Can you work these out from the model? Positions are in its coordinate system, mm. Give positions to 0.01 mm unless a question says otherwise; leave off trailing zeros. Order: outer loops, then holes, each group sorted by start corner. A loop starts at its lowest first (then second) coordinate and runs counter-clockwise, first axis right, second up. Notation, with made-up numbers: (44.5, 83) - (54.5, 83) arc R22 ccw to (54.5, 97) - close; hole circle Ø3 at (87.25, 3). An arc over 180 degrees is marked (long way). Return JSON: item names as keys, results as strings.
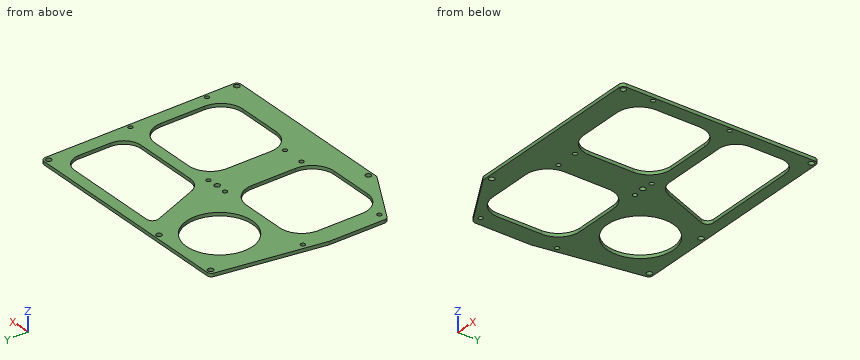
```python
from build123d import *

# Parameters (mm, degrees)
SKETCH_R   = 2.5
SKETCH_R_2 = 2
SKETCH_R_3 = 30.106081
PAD_DEPTH  = 3
FILLET_R   = 4


with BuildPart() as part:
    # Sketch → Pad (new body)
    with BuildSketch(Plane.XY.offset(30)):
        Polygon((162.56, -90.17), (-5.000233, -90.169747), (-56.898089, -60.365632), (-56.898089, -7.158878), (-41.241165, 90.17), (162.56, 90.17), align=None)
        with Locations((25.4, 86.106)):
            Circle(SKETCH_R, mode=Mode.SUBTRACT)
        with Locations((158.496, 86.106)):
            Circle(SKETCH_R, mode=Mode.SUBTRACT)
        with Locations((55.4, 10.106)):
            Circle(SKETCH_R, mode=Mode.SUBTRACT)
        with Locations((0.007, -86.11)):
            Circle(SKETCH_R, mode=Mode.SUBTRACT)
        with Locations((158.496, -86.106)):
            Circle(SKETCH_R, mode=Mode.SUBTRACT)
        with Locations((-36.83, 86.11)):
            Circle(SKETCH_R, mode=Mode.SUBTRACT)
        with Locations((159.06, -59.17)):
            Circle(SKETCH_R_2, mode=Mode.SUBTRACT)
        with Locations((159.059998, 10.83)):
            Circle(SKETCH_R_2, mode=Mode.SUBTRACT)
        with Locations((65.059998, 10.830006)):
            Circle(SKETCH_R_2, mode=Mode.SUBTRACT)
        with Locations((65.06, -59.169994)):
            Circle(SKETCH_R_2, mode=Mode.SUBTRACT)
        with Locations((45.06, -59.169992)):
            Circle(SKETCH_R_2, mode=Mode.SUBTRACT)
        with Locations((45.059997, 10.830008)):
            Circle(SKETCH_R_2, mode=Mode.SUBTRACT)
        with Locations((-48.940003, 10.830015)):
            Circle(SKETCH_R_2, mode=Mode.SUBTRACT)
        with Locations((-48.94, -59.169984)):
            Circle(SKETCH_R_2, mode=Mode.SUBTRACT)
        with Locations((0, 50)):
            Circle(SKETCH_R_3, mode=Mode.SUBTRACT)
        with BuildLine():
            ThreePointArc((90.000007, 10), (75.857866, 4.142134), (70, -10.000007))
            Line((70, -50), (70, -10.000007))
            ThreePointArc((70, -50), (75.857866, -64.14214), (90.000007, -70.000007))
            Line((130, -70.000007), (90.000007, -70.000007))
            ThreePointArc((130, -70.000007), (144.14214, -64.14214), (150.000007, -50))
            Line((150.000007, -10.000007), (150.000007, -50))
            ThreePointArc((150.000007, -10.000007), (144.14214, 4.142134), (130, 10))
            Line((90.000007, 10), (130, 10))
        make_face(mode=Mode.SUBTRACT)
        with BuildLine():
            Line((-40, -50.00001), (-40, -10.000017))
            ThreePointArc((-19.999993, 9.99999), (-34.142134, 4.142124), (-40, -10.000017))
            Line((-19.999993, 9.99999), (20, 9.99999))
            ThreePointArc((40.000007, -10.000017), (34.14214, 4.142124), (20, 9.99999))
            Line((40.000007, -10.000017), (40.000007, -50.00001))
            ThreePointArc((20, -70.000017), (34.14214, -64.14215), (40.000007, -50.00001))
            Line((20, -70.000017), (-19.999993, -70.000017))
            ThreePointArc((-40, -50.00001), (-34.142134, -64.14215), (-19.999993, -70.000017))
        make_face(mode=Mode.SUBTRACT)
        with BuildLine():
            ThreePointArc((134.197919, 20), (145.371681, 24.628324), (150.000005, 35.802086))
            Line((150.000005, 65.000005), (150.000005, 35.802086))
            ThreePointArc((150.000005, 65.000005), (145.606605, 75.606611), (135, 80.00001))
            Line((48.267642, 80.00001), (135, 80.00001))
            ThreePointArc((48.267642, 80.00001), (43.934723, 77.707276), (43.393027, 72.835172))
            Line((60.301612, 30.000089), (43.393027, 72.835172))
            ThreePointArc((60.301612, 30.000089), (66.111185, 22.737064), (75.000005, 20))
            Line((134.197919, 20), (75.000005, 20))
        make_face(mode=Mode.SUBTRACT)
    extrude(amount=PAD_DEPTH)

    # Fillet
    fillet_edges = [part.edges().sort_by_distance(p)[0] for p in [
        (-5.000233, -90.169747, 31.5),
        (162.56, -90.17, 31.5),
        (162.56, 90.17, 31.5),
        (-56.898089, -60.365632, 31.5),
        (-56.898089, -7.158878, 31.5),
        (-41.241165, 90.17, 31.5),
    ]]
    fillet(fillet_edges, radius=FILLET_R)


solid = part.part
```
1. Suppose I cut it at B-B (x = -22.5). List the corners of the cut face in (y, z) for me.
Checks:
{"outline": "(-80.12, 30) - (-69.84, 30) - (-69.84, 33) - (-80.12, 33) - close; (9.84, 30) - (30, 30) - (30, 33) - (9.84, 33) - close; (70, 30) - (90.17, 30) - (90.17, 33) - (70, 33) - close"}
2. For pin 1 Ø3 at (x, y) = (45.06, -59.17) entering from +Z; pin 2 Ø5 at (x, y) = (45.06, 10.83) entering from +Z, each with a flat end and sliding along its axis, tell me the tip position at first contact or that it passes through.
Checks:
{"pin 1": "through", "pin 2": "z = 33"}
3. Suppose I cut it at C-C (z = 31.9). State how many separate pieces and enclosed holes the cut face has, plus the area to 3 significant figures.
Checks:
{"separate pieces": "1", "enclosed holes": "18", "area": "17,100 mm^2"}
4. If I drill on L1, parallel to Y at x = 124.5, z = 32.35; L2, parallel to Y at x = 0, z = 31.35; L3, parallel to X at y = -46, z = 32.7, over which ranges is the centre line in solid material (lowest first)? Write a range as [from, to].
Checks:
{"L1": "[-90.17, -70], [10, 20], [80, 90.17]", "L2": "[-90.17, -88.61], [-83.61, -70], [10, 19.89], [80.11, 90.17]", "L3": "[-56.9, -40], [40, 70], [150, 162.56]"}
5. Suppose I cut it at A-A (y = -36.5). List the corners of the cut face in (x, z) for me, plus the area to 3 significant figures.
Checks:
{"outline": "(-56.9, 30) - (-40, 30) - (-40, 33) - (-56.9, 33) - close; (40, 30) - (70, 30) - (70, 33) - (40, 33) - close; (150, 30) - (162.56, 30) - (162.56, 33) - (150, 33) - close", "area": "178 mm^2"}
